The drawing under review shows one solid part. Ordinate dimensions are in mm from its lowest x, y, z. A direction names the side the tool comes from. Coordinates: 2 decimals unless noted, no trailing zeros. Order: outer loops, then holes, each group sorted by start corner. A loop starts at its lowest first (then second) coordinate and runs counter-clockwise, first axis right, second up. Notation, with made-up numbers: (-12, -25.5) -> (34, -25.5) arc R22 ccw to (34, 2.5) -> close; hole circle Ø2 at (-35, 81). An arc over 180 degrees is marked (long way). Write item = value, one per line.
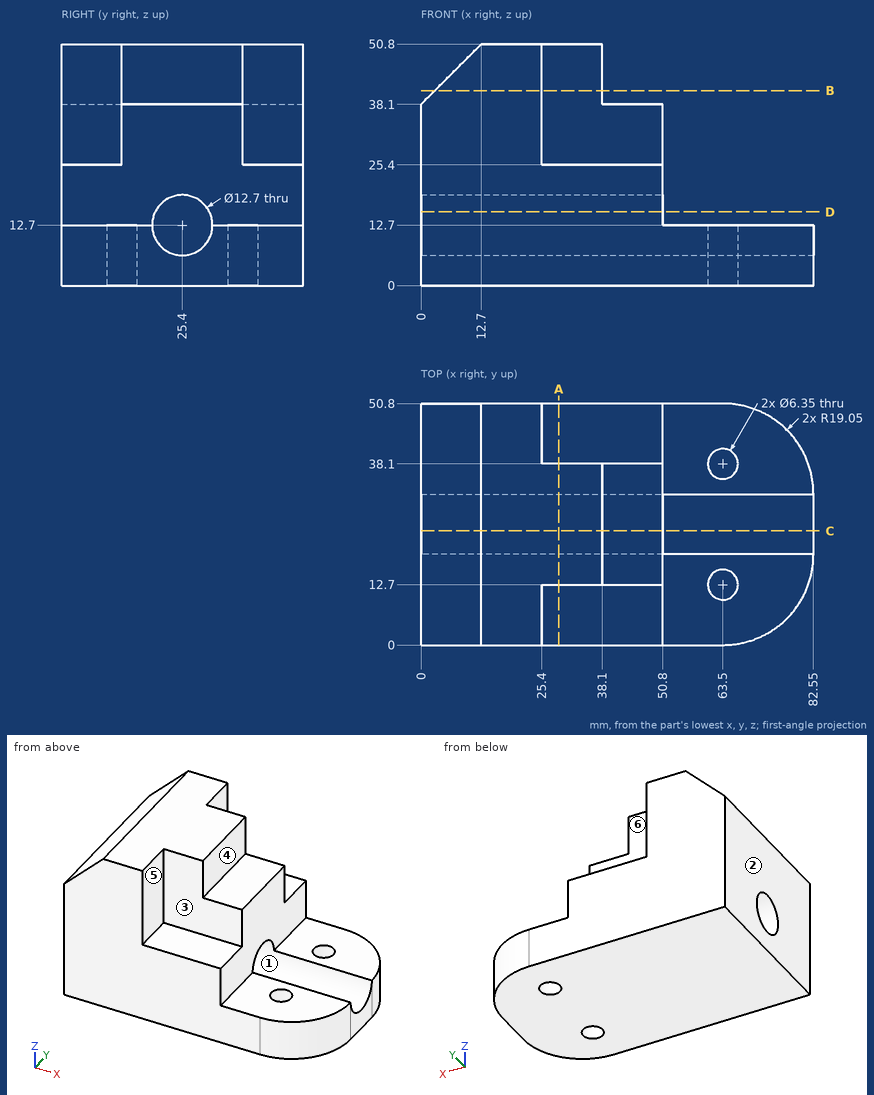
(1) We need section B-B (z = 41). Write out the cut boundary in (x, y), and give its area (3 significant figures).
Report:
outline = (2.9, 0) -> (25.4, 0) -> (25.4, 12.7) -> (38.1, 12.7) -> (38.1, 38.1) -> (25.4, 38.1) -> (25.4, 50.8) -> (2.9, 50.8) -> close
area = 1,470 mm²
(2) The part is to be moulded in two halves that separate along Y. For the marked faces 1, 2 and 3, say which applies: released by +Y, released by -Y, zero draft, split by the parting line, or undercut.
Report:
face_1 = undercut
face_2 = zero draft
face_3 = released by -Y
(3) Insertion check: pin 1 (14 mm diameter, centred on y = 3.5, z = 35.5, fed in from +X); pin 2 (14 mm diameter, centred on x = 45.5, y = 27, fed in from +Z); pin 3 (14 mm diameter, centred on x = 36, y = 4.5, fed in from +Z); pin 4 (8 mm diameter, centred on x = 49.5, y = 21, fed in from -Z). Each pin has a flat end and moves straight along its axis. Give the tip position at first contact, or say it passes through.
Report:
pin_1 = 25.4
pin_2 = 38.1
pin_3 = 25.4
pin_4 = 0
(4) For the marked faces 4, 5 and 6, list the 3-axis set-ups (+Z, -Z, +X, -X, +Y, -Y) from which the entire face can be reached by the end or side of a thin tool; tool diameter is ignored.
Report:
face_4 = +Z, +X, +Y, -Y
face_5 = +Z, +X, -Y
face_6 = +Z, +X, +Y
(5) We need section C-C (y = 24). Write out the cut boundary in (x, z), and give its area (3 significant figures).
Report:
outline = (0, 0) -> (82.55, 0) -> (82.55, 6.51) -> (0, 6.51) -> close; (0, 18.89) -> (50.8, 18.89) -> (50.8, 38.1) -> (38.1, 38.1) -> (38.1, 50.8) -> (12.7, 50.8) -> (0, 38.1) -> close
area = 1,920 mm²
(6) We need section A-A (x = 29). Write out the cut boundary in (y, z).
Report:
outline = (0, 0) -> (50.8, 0) -> (50.8, 25.4) -> (38.1, 25.4) -> (38.1, 50.8) -> (12.7, 50.8) -> (12.7, 25.4) -> (0, 25.4) -> close; hole circle Ø12.7 at (25.4, 12.7)
(7) We need section D-D (z = 15.5). Write out the cut boundary in (x, y).
Report:
outline = (0, 0) -> (50.8, 0) -> (50.8, 19.7) -> (0, 19.7) -> close; (0, 31.1) -> (50.8, 31.1) -> (50.8, 50.8) -> (0, 50.8) -> close
(8) For L1, parallel to Y at x = 32, z = 12.7; L2, parallel to Y at x = 65, z = 4; L3, parallel to X at y = 3, z = 15.5, list the stretches that pass through material, from the lowest coordinate up.
Report:
L1 = 0 to 19.05, 31.75 to 50.8
L2 = 0.06 to 9.9, 15.5 to 35.3, 40.9 to 50.74
L3 = 0 to 50.8
